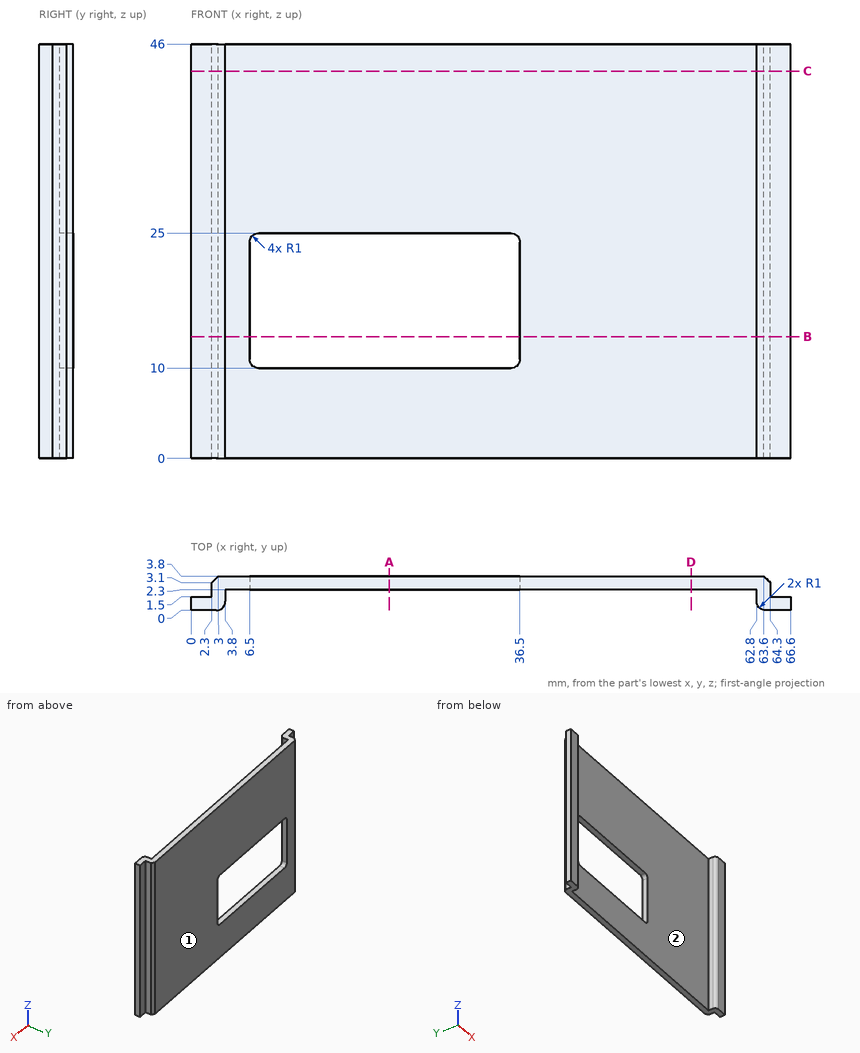
Input: dimensioned drawing with shaded views. Units: mm. Origin: part minimum x, y, z. Round coordinates to 2 decimals unless told otherwise and drop trailing zeros. Order: outer loops, then holes, each group sorted by start corner. A loop starts at its lowest first (then second) coordinate and runs counter-clockwise, first axis right, second up.
Q1. Pin query (flat end, axial travel): pin 1 (0.7 mm diameter, centred on x = 65, z = 29.5, fed in from +Y); pin 2 (0.5 mm diameter, centred on y = 3, z = 18.5, fed in from +X); pin 3 (1.8 mm diameter, centred on y = 2.5, z = 15.5, fed in from -X). Return the tip coordinate at first contact, or that it passes through.
Result sheet:
pin 1: stops at y = 1.5
pin 2: stops at x = 64.3
pin 3: stops at x = 2.3
Q2. Material intervals for probe 1 along X at (y, z) = (2, 33.5); probe 2 along Z at (x, y) = (23, 2.7); probe 3 along X at (y, z) = (0.85, 4), sorted ascending.
Result sheet:
probe 1: x = 2.3 to 3.8, 62.8 to 64.3
probe 2: z = 0 to 10, 25 to 46
probe 3: x = 0 to 3.79, 62.81 to 66.6
Q3. Mould query, pull axis X, two halves, no side actions, for the marked faces 1 and 2. Classes: released by +X, released by -X, zero draft, split by the parting line, or undercut.
Result sheet:
face 1: zero draft
face 2: undercut
Q4. Section B-B, the plane z = 13.5. Output: boundary loops of the cut face in (x, y).
Result sheet:
outline: (0, 0) - (2.8, 0) arc R1 ccw to (3.8, 1) - (3.8, 2.3) - (6.5, 2.3) - (6.5, 3.8) - (3, 3.8) - (2.3, 3.1) - (2.3, 1.5) - (0, 1.5) - close; (36.5, 2.3) - (62.8, 2.3) - (62.8, 1) arc R1 ccw to (63.8, 0) - (66.6, 0) - (66.6, 1.5) - (64.3, 1.5) - (64.3, 3.1) - (63.6, 3.8) - (36.5, 3.8) - close
Q5. Section C-C, the plane z = 43. Output: boundary loops of the cut face in (x, y), and give its area (3 significant figures).
Result sheet:
outline: (0, 0) - (2.8, 0) arc R1 ccw to (3.8, 1) - (3.8, 2.3) - (62.8, 2.3) - (62.8, 1) arc R1 ccw to (63.8, 0) - (66.6, 0) - (66.6, 1.5) - (64.3, 1.5) - (64.3, 3.1) - (63.6, 3.8) - (3, 3.8) - (2.3, 3.1) - (2.3, 1.5) - (0, 1.5) - close
area: 106 mm2
Q6. Section D-D, the plane x = 55.5. Output: boundary loops of the cut face in (y, z), and give its area (3 significant figures).
Result sheet:
outline: (2.3, 0) - (3.8, 0) - (3.8, 46) - (2.3, 46) - close
area: 69.0 mm2
Q7. Section A-A, the plane x = 22. Output: boundary loops of the cut face in (y, z).
Result sheet:
outline: (2.3, 0) - (3.8, 0) - (3.8, 10) - (2.3, 10) - close; (2.3, 25) - (3.8, 25) - (3.8, 46) - (2.3, 46) - close
